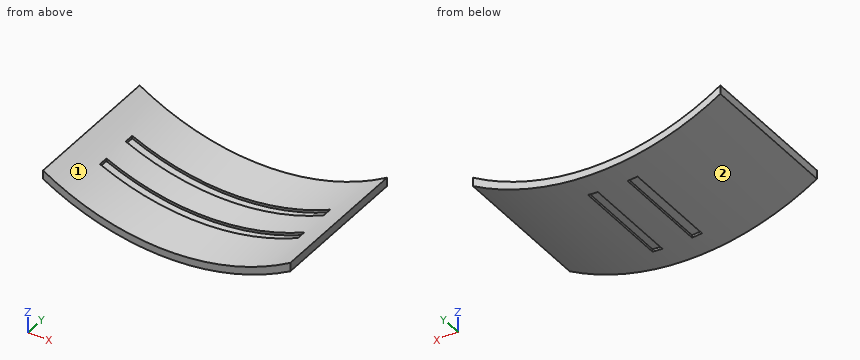
```python
from build123d import *

# Parameters (mm, degrees)
BOSS_EXTRUDE1_DEPTH      = 30
CUT_EXTRUDE28_REACH      = 65.05
CUT_EXTRUDE28_END_RADIUS = 48.5
SKETCH3_W                = 40
SKETCH3_H                = 2
CUT_EXTRUDE29_REACH      = 45.439
CUT_EXTRUDE29_END_RADIUS = 49
SKETCH5_W                = 2
SKETCH5_H                = 20


with BuildPart() as part:
    # Sketch2 → Boss-Extrude1 (new body)
    with BuildSketch(Plane(origin=(0, 0, 0), x_dir=(1, 0, 0), z_dir=(0, 1, 0))):
        with BuildLine():
            Line((-25, 42.722944655), (-25, 40.975602497))
            ThreePointArc((-25, 40.975602497), (0, 48), (25, 40.975602497))
            Line((25, 40.975602497), (25, 42.722944655))
            ThreePointArc((25, 42.722944655), (0, 49.5), (-25, 42.722944655))
        make_face()
    extrude(amount=BOSS_EXTRUDE1_DEPTH)

    # Cut-Extrude28: up to this cylinder (the profile starts inside it)
    cut_extrude28_end = Plane(origin=(0, 15, 0), z_dir=(0, -1, 0)) * Cylinder(CUT_EXTRUDE28_END_RADIUS, 236.1, mode=Mode.PRIVATE)
    # Sketch3 → Cut-Extrude28 (cut, up to the surface)
    with BuildSketch(Plane(origin=(0, 0, 0), x_dir=(-1, 0, 0), z_dir=(0, 0, -1)), mode=Mode.PRIVATE) as cut_extrude28_sk1:
        with Locations((0, 19)):
            Rectangle(SKETCH3_W, SKETCH3_H)
    cut_extrude28_tool1 = extrude(cut_extrude28_sk1.sketch, amount=CUT_EXTRUDE28_REACH, mode=Mode.PRIVATE) & cut_extrude28_end
    add(cut_extrude28_tool1.solids().sort_by_distance((0, 19, 0))[0], mode=Mode.SUBTRACT)
    # Sketch3 → Cut-Extrude28 (cut, up to the surface)
    with BuildSketch(Plane(origin=(0, 0, 0), x_dir=(-1, 0, 0), z_dir=(0, 0, -1)), mode=Mode.PRIVATE) as cut_extrude28_sk2:
        with Locations((0, 11)):
            Rectangle(SKETCH3_W, SKETCH3_H)
    cut_extrude28_tool2 = extrude(cut_extrude28_sk2.sketch, amount=CUT_EXTRUDE28_REACH, mode=Mode.PRIVATE) & cut_extrude28_end
    add(cut_extrude28_tool2.solids().sort_by_distance((0, 11, 0))[0], mode=Mode.SUBTRACT)

    # Cut-Extrude29: up to this cylinder (the profile starts outside it)
    cut_extrude29_end = Plane(origin=(0, 15, 0), z_dir=(0, -1, 0)) * Cylinder(CUT_EXTRUDE29_END_RADIUS, 189.878, mode=Mode.PRIVATE)
    # Sketch5 → Cut-Extrude29 (cut, up to the surface)
    with BuildSketch(Plane.XY.offset(-60), mode=Mode.PRIVATE) as cut_extrude29_sk1:
        with Locations((-4, 15)):
            Rectangle(SKETCH5_W, SKETCH5_H)
    cut_extrude29_tool1 = extrude(cut_extrude29_sk1.sketch, amount=CUT_EXTRUDE29_REACH, mode=Mode.PRIVATE) - cut_extrude29_end
    add(cut_extrude29_tool1.solids().sort_by_distance((-4, 15, -60))[0], mode=Mode.SUBTRACT)
    # Sketch5 → Cut-Extrude29 (cut, up to the surface)
    with BuildSketch(Plane.XY.offset(-60), mode=Mode.PRIVATE) as cut_extrude29_sk2:
        with Locations((4, 15)):
            Rectangle(SKETCH5_W, SKETCH5_H)
    cut_extrude29_tool2 = extrude(cut_extrude29_sk2.sketch, amount=CUT_EXTRUDE29_REACH, mode=Mode.PRIVATE) - cut_extrude29_end
    add(cut_extrude29_tool2.solids().sort_by_distance((4, 15, -60))[0], mode=Mode.SUBTRACT)


solid = part.part
```
Source: CAD feature listing. Evaluate the final solid. Frame: model axes, mm. Face numbers are marked on the shaded views. Coordinates: 2 decimals unless noted, no trailing zeros. Write each loop counter-clockwise with the first axis right and the second up, starting at its lowest first coordinate (ties: lowest second). Pieces come first, ordered by that corner, then holes. Notation, with made-up numbers: (-33.5, -8.75) -> (-10.5, -8.75) arc R27 ccw to (-10.5, 16.25) -> close; hole circle Ø8 at (85, -37). An arc over 180 degrees is marked (long way). Return JSON: item names as keys, results as strings. Group by question number.
1) Mould query, pull axis X, two halves, no side actions, for the marked faces 1 and 2. Classes: +X half, -X half, draft (parallel to the pull), parting line (faces both ways), or undercut.
2) Section query C-C, the plane x = -1.5. Return loops of the section in (y, z).
3) Section query D-D, the plane y = 23. Return loops of the section in (x, z).
4) Section query A-A, the plane y = 10.5. Return loops of the section in (x, z).
5) Section query B-B, the plane z = -45.5. Return loops of the section in (x, y), plus the area to 3 significant figures.
6) Ray query, line 1 along X through (y, z) = (19, -44.5); line 2 along X through (y, z) = (13.75, -44); line 3 along Z through (x, y) = (1.5, 21.75). Return the intervals inside material, ascending.
7) Contact query for flat-ended pins moving along their axis: P1, Ø4, axis at x = -3.5, y = 10.5, coming from the -Z side; P2, Ø1.5, axis at x = 15, y = 6, coming from the -Z side; P3, Ø1.5, axis at x = -14.5, y = 21.5, coming from the -Z side. Output: stop coordinate, or through.
From the geometry:
{
 "1": {"face 1": "undercut", "face 2": "parting line"},
 "2": {"outline": "(0, -49.48) -> (30, -49.48) -> (30, -47.98) -> (20, -47.98) -> (20, -48.48) -> (18, -48.48) -> (18, -47.98) -> (12, -47.98) -> (12, -48.48) -> (10, -48.48) -> (10, -47.98) -> (0, -47.98) -> close"},
 "3": {"outline": "(-25, -42.72) arc R49.5 ccw to (-5, -49.25) -> (-5, -48.74) arc R49 ccw to (-3, -48.91) -> (-3, -49.41) arc R49.5 ccw to (3, -49.41) -> (3, -48.91) arc R49 ccw to (5, -48.74) -> (5, -49.25) arc R49.5 ccw to (25, -42.72) -> (25, -40.98) arc R48 cw to (-25, -40.98) -> close"},
 "4": {"outline": "(-25, -42.72) arc R49.5 ccw to (-5, -49.25) -> (-5, -48.74) arc R49 ccw to (-3, -48.91) -> (-3, -49.41) arc R49.5 ccw to (3, -49.41) -> (3, -48.91) arc R49 ccw to (5, -48.74) -> (5, -49.25) arc R49.5 ccw to (25, -42.72) -> (25, -40.98) arc R48 cw to (20, -43.63) -> (20, -44.18) arc R48.5 cw to (-20, -44.18) -> (-20, -43.63) arc R48 cw to (-25, -40.98) -> close"},
 "5": {"outline": "(-19.49, 0) -> (-15.29, 0) -> (-15.29, 10) -> (-16.79, 10) -> (-16.79, 12) -> (-15.29, 12) -> (-15.29, 18) -> (-16.79, 18) -> (-16.79, 20) -> (-15.29, 20) -> (-15.29, 30) -> (-19.49, 30) -> close; (15.29, 0) -> (19.49, 0) -> (19.49, 30) -> (15.29, 30) -> (15.29, 20) -> (16.79, 20) -> (16.79, 18) -> (15.29, 18) -> (15.29, 12) -> (16.79, 12) -> (16.79, 10) -> (15.29, 10) -> close", "area": "240 mm²"},
 "6": {"line 1": "-21.68 to -19.29, 19.29 to 21.68", "line 2": "-22.68 to -19.18, 19.18 to 22.68", "line 3": "-49.48 to -47.98"},
 "7": {"P1": "z = -49.48", "P2": "z = -47.4", "P3": "z = -47.55"}
}
